```python
from build123d import *

# Parameters (mm, degrees)
BOSS_EXTRUDE1_DEPTH              = 11.1252
F_1_4_20_TAPPED_HOLE1_AT_2_COUNT = 2
F_1_4_20_TAPPED_HOLE1_AT_2_PITCH = 101.6
F_1_4_20_TAPPED_HOLE1_AT_3_COUNT = 2
F_1_4_20_TAPPED_HOLE1_AT_3_PITCH = 49.130736385
F_1_4_20_TAPPED_HOLE2_AT_2_COUNT = 2
F_1_4_20_TAPPED_HOLE2_AT_2_PITCH = 53.975
F_1_4_20_TAPPED_HOLE2_AT_3_COUNT = 2
F_1_4_20_TAPPED_HOLE2_AT_3_PITCH = 111.125
F_1_4_20_TAPPED_HOLE2_AT_4_COUNT = 2
F_1_4_20_TAPPED_HOLE2_AT_4_PITCH = 49.1998
CUT_EXTRUDE1_DEPTH               = 12.1252001
CHAMFER3_SIZE                    = 3.175
CUT_EXTRUDE2_DEPTH               = 119.608154476
CUT_EXTRUDE3_DEPTH               = 12.1252001
F_1_8_0_125_DIAMETER_HOLE1_D     = 3.175
CUT_EXTRUDE4_DEPTH               = 12.1252001


with BuildPart() as part:
    # Sketch1 → Boss-Extrude1 (new body)
    with BuildSketch(Plane.XY):
        Polygon((0, 0), (0, -182.6405415), (118.608154476, 0), align=None)
        with BuildLine():
            Line((19.802154476, -13.462), (82.118989682, -13.462))
            ThreePointArc((82.118989682, -13.462), (87.699478347, -16.782041872), (87.444547788, -23.270457872))
            Line((87.444547788, -23.270457872), (25.127712583, -119.229969062))
            ThreePointArc((25.127712583, -119.229969062), (17.998657037, -121.860016506), (13.452154476, -115.771511189))
            Line((13.452154476, -115.771511189), (13.452154476, -19.812))
            ThreePointArc((13.452154476, -19.812), (15.312026416, -15.321871939), (19.802154476, -13.462))
        make_face(mode=Mode.SUBTRACT)
    extrude(amount=BOSS_EXTRUDE1_DEPTH)

    # Sketch3 → 1/4-20 Tapped Hole1 (revolve, cut)
    with BuildSketch(Plane(origin=(0, -139.805902277, 5.5626), x_dir=(0, 0, 1), z_dir=(0, 1, 0))):
        Polygon((0, 0), (0, 32.217016902), (2.5527, 30.6832), (2.5527, 15.24), (3.175, 15.24), (3.175, 0.889), (4.064, 0), align=None)
    f_1_4_20_tapped_hole1 = revolve(axis=Axis((-6.35, -139.805902277, 5.5626), (1, 0, 0)), mode=Mode.SUBTRACT)

    # 1/4-20 Tapped Hole1 at 2: 1/4-20 Tapped Hole1 ×2
    with Locations(*[(0, i * F_1_4_20_TAPPED_HOLE1_AT_2_PITCH, 0) for i in range(1, F_1_4_20_TAPPED_HOLE1_AT_2_COUNT)]):
        add(f_1_4_20_tapped_hole1, mode=Mode.SUBTRACT)

    # 1/4-20 Tapped Hole1 at 3: 1/4-20 Tapped Hole1 ×2
    with Locations(*[(0, i * F_1_4_20_TAPPED_HOLE1_AT_3_PITCH, 0) for i in range(1, F_1_4_20_TAPPED_HOLE1_AT_3_COUNT)]):
        add(f_1_4_20_tapped_hole1, mode=Mode.SUBTRACT)

    # Sketch6 → 1/4-20 Tapped Hole2 (revolve, cut)
    with BuildSketch(Plane(origin=(74.349919226, -68.151705822, 5.5626), x_dir=(0.544639035, 0.838670568, 0), z_dir=(0, 0, 1))):
        Polygon((0, 0), (0, 19.517016902), (2.5527, 17.9832), (2.5527, 15.24), (3.175, 15.24), (3.175, 0.889), (4.064, 0), align=None)
    f_1_4_20_tapped_hole2 = revolve(axis=Axis((79.675477332, -71.610163694, 5.5626), (-0.838670568, 0.544639035, 0)), mode=Mode.SUBTRACT)

    # 1/4-20 Tapped Hole2 at 2: 1/4-20 Tapped Hole2 ×2
    with Locations(*[Vector(-0.544639035, -0.838670568, 0) * (i * F_1_4_20_TAPPED_HOLE2_AT_2_PITCH) for i in range(1, F_1_4_20_TAPPED_HOLE2_AT_2_COUNT)]):
        add(f_1_4_20_tapped_hole2, mode=Mode.SUBTRACT)

    # 1/4-20 Tapped Hole2 at 3: 1/4-20 Tapped Hole2 ×2
    with Locations(*[Vector(-0.544639035, -0.838670568, 0) * (i * F_1_4_20_TAPPED_HOLE2_AT_3_PITCH) for i in range(1, F_1_4_20_TAPPED_HOLE2_AT_3_COUNT)]):
        add(f_1_4_20_tapped_hole2, mode=Mode.SUBTRACT)

    # 1/4-20 Tapped Hole2 at 4: 1/4-20 Tapped Hole2 ×2
    with Locations(*[Vector(0.544639035, 0.838670568, 0) * (i * F_1_4_20_TAPPED_HOLE2_AT_4_PITCH) for i in range(1, F_1_4_20_TAPPED_HOLE2_AT_4_COUNT)]):
        add(f_1_4_20_tapped_hole2, mode=Mode.SUBTRACT)

    # Sketch8 → Cut-Extrude1 (cut, through all)
    with BuildSketch(Plane.XY.offset(11.1252)):
        Polygon((0, -182.6405415), (0, -173.1155415), (6.185607325, -173.1155415), align=None)
    extrude(amount=-CUT_EXTRUDE1_DEPTH, mode=Mode.SUBTRACT)

    # Chamfer3
    chamfer3_edges = [part.edges().sort_by_distance(p)[0] for p in [
        (0, 0, 5.5626),
    ]]
    chamfer(chamfer3_edges, length=CHAMFER3_SIZE)

    # Sketch9 → Cut-Extrude2 (cut, through all)
    with BuildSketch(Plane.ZY):
        Polygon((11.1252, 0), (0, 0), (0, -0.973328879), align=None)
    extrude(amount=-CUT_EXTRUDE2_DEPTH, mode=Mode.SUBTRACT)

    # Sketch10 → Cut-Extrude3 (cut, through all)
    with BuildSketch(Plane.XY.offset(11.1252)):
        Polygon((118.608154476, 0), (116.322154476, 0), (116.322154476, -3.520131307), align=None)
    extrude(amount=-CUT_EXTRUDE3_DEPTH, mode=Mode.SUBTRACT)

    # 1/8 (0.125) Diameter Hole1 (through all)
    with Locations(Plane.XY.offset(11.1252)):
        with Locations((16.8148, -139.805902277)):
            Hole(F_1_8_0_125_DIAMETER_HOLE1_D / 2)

    # Sketch14 → Cut-Extrude4 (cut, through all)
    with BuildSketch(Plane.XY.offset(11.1252)):
        Polygon((0, -150.3825415), (0, -152.6685415), (1.143, -151.5255415), align=None)
    extrude(amount=-CUT_EXTRUDE4_DEPTH, mode=Mode.SUBTRACT)


solid = part.part
```
Read the model definition and answer for the solid it produces. Units are mm, in the model's axes. A direction names the side the tool comes from. Give positions to 0.01 mm unless a question says otherwise; leave off trailing zeros. Order: outer loops, then holes, each group sorted by start corner. A loop starts at its lowest first (then second) coordinate and runs counter-clockwise, first axis right, second up.
(1) For a pull along X with two mould halves and no side action, classify faces 6 (the cylindrical face through (37.28, -112.22, 5.42)), 7 (the conical face through (44, -114, 9)), 8 (the flat face through (0, -163, 5)), 9 (the flat face through (3, -173.116, 6)) as released by +X, released by -X, zero draft, split by the parting line, or undercut.
(2) Given pin 1 (1.5 mm diameter, centred on y = -141, z = 4.5, fed in from -X); pin 2 (5.5 mm diameter, centred on x = 39, z = 4, fed in from -Y); pin 3 (4 mm diameter, centred on y = -38.21, z = 5.56, fed in from +X); pin 4 (3.5 mm diameter, centred on x = 16.81, y = -139.81, fed in from +Z), each flat-ended and moving along its own axis, determine where each tip first touches the part or whether it passes through.
(3) Find section A-A (y = -55). Give the vertices of the cut face in (x, z).
(4) Find section B-B (y = -132). Give the vertices of the cut face in (x, z).
(5) Straight lines are drawn through the part: L1, parallel to Y at x = 10.5, z = 6; L2, parallel to Y at x = 20.5, z = 4.75; L3, parallel to X at y = -95, z = 4.5. For each, find the intervals that lie inside material, in ascending order.
(6) For faces 1 (the cylindrical face through (7.964, -142.954, 5.149)), 2 (the cylindrical face through (15.263, -15.372, 5.485)), 3 (the flat face through (58.463, -0.493, 5.485)), 4 (the flat face through (1.257, -1.918, 5.485)), 5 (the flat face through (2.524, -150.772, 5.783)), determine the directions among +Z, -Z, +X, -X, +Y, -Y from which every point of the face is accessible in a straight line to the end or side of a thin tool.
Result sheet:
1. face 6: undercut
1. face 7: released by +X
1. face 8: released by -X
1. face 9: zero draft
2. pin 1: passes through
2. pin 2: stops at y = -126.82
2. pin 3: stops at x = 95.09
2. pin 4: stops at z = 11.13
3. outline: (0, 0) - (13.45, 0) - (13.45, 11.13) - (0, 11.13) - close; (66.84, 0) - (82.89, 0) - (82.89, 11.13) - (66.84, 11.13) - close
4. outline: (0, 0) - (32.89, 0) - (32.89, 11.13) - (0, 11.13) - close
5. L1: y = -166.47 to -162.94, -155.44 to -142.95, -136.66 to -93.82, -87.53 to -41.35, -35.06 to -0.45
5. L2: y = -151.07 to -142.23, -137.39 to -122.08, -13.46 to -0.56
5. L3: x = 0 to 13.45, 40.86 to 56.91
6. face 1: -X
6. face 2: +Z, -Z
6. face 3: -Z, +X, -X, +Y
6. face 4: +Z, -Z, -X, +Y
6. face 5: none
